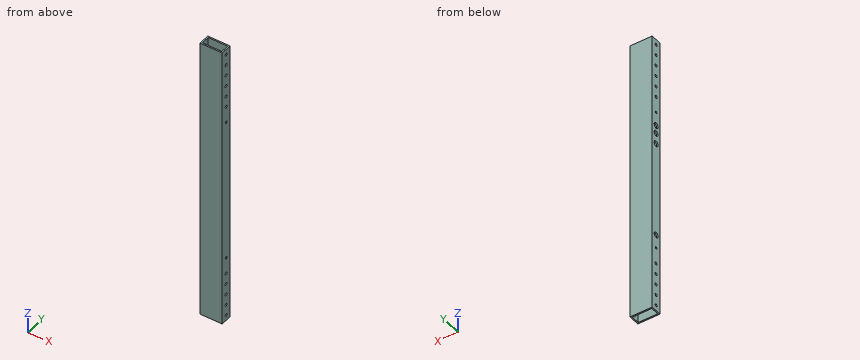
from build123d import *

# Parameters (mm, degrees)
BOSS_EXTRUDE1_DEPTH              = 330.2
BOSS_EXTRUDE1_DEPTH_BACK         = 330.2
SKETCH3_W                        = 50.8
SKETCH3_H                        = 25.4
SKETCH3_W_2                      = 44.45
SKETCH3_H_2                      = 19.05
F_1_4_0_25_DIAMETER_HOLE3_D      = 6.35
F_1_4_0_25_DIAMETER_HOLE4_D      = 6.35
F_1_4_0_25_DIAMETER_HOLE5_D      = 6.35
F_1_4_0_25_DIAMETER_HOLE6_D      = 6.35
F_1_4_0_25_DIAMETER_HOLE7_D      = 6.35
F_1_4_0_25_DIAMETER_HOLE8_D      = 6.35
F_13_64_0_20313_DIAMETER_HOLE1_D = 5.159502
F_1_2_0_5_DIAMETER_HOLE1_D       = 12.7
F_1_2_0_5_DIAMETER_HOLE1_DEPTH   = 6.35
F_1_2_0_5_DIAMETER_HOLE1_TIP     = 3.815464931


with BuildPart() as part:
    # Sketch3 → Boss-Extrude1 (new, two sides: drawn at the far end of the back side and taken through both)
    with BuildSketch(Plane.XY.offset(-BOSS_EXTRUDE1_DEPTH_BACK)):
        Rectangle(SKETCH3_W, SKETCH3_H)
        Rectangle(SKETCH3_W_2, SKETCH3_H_2, mode=Mode.SUBTRACT)
    extrude(amount=BOSS_EXTRUDE1_DEPTH + BOSS_EXTRUDE1_DEPTH_BACK)

    # 1/4 (0.25) Diameter Hole3 (through all)
    with Locations(Plane.ZY.offset(25.4)):
        with Locations((-317.5, 0)):
            Hole(F_1_4_0_25_DIAMETER_HOLE3_D / 2)

    # 1/4 (0.25) Diameter Hole4 (through all)
    with Locations(Plane.ZY.offset(25.4)):
        with Locations((292.1, 0), (317.5, 0)):
            Hole(F_1_4_0_25_DIAMETER_HOLE4_D / 2)

    # 1/4 (0.25) Diameter Hole5 (through all)
    with Locations(Plane(origin=(25.4, 0, 0), x_dir=(0, 0, -1), z_dir=(1, 0, 0))):
        with Locations((292.1, 0), (266.7, 0)):
            Hole(F_1_4_0_25_DIAMETER_HOLE5_D / 2)

    # 1/4 (0.25) Diameter Hole6 (through all)
    with Locations(Plane(origin=(25.4, 0, 0), x_dir=(0, 0, -1), z_dir=(1, 0, 0))):
        with Locations((215.9, 0), (241.3, 0)):
            Hole(F_1_4_0_25_DIAMETER_HOLE6_D / 2)

    # 1/4 (0.25) Diameter Hole7 (through all)
    with Locations(Plane(origin=(25.4, 0, 0), x_dir=(0, 0, -1), z_dir=(1, 0, 0))):
        with Locations((-190.5, 0), (-215.9, 0)):
            Hole(F_1_4_0_25_DIAMETER_HOLE7_D / 2)

    # 1/4 (0.25) Diameter Hole8 (through all)
    with Locations(Plane(origin=(25.4, 0, 0), x_dir=(0, 0, -1), z_dir=(1, 0, 0))):
        with Locations((-266.7, 0), (-241.3, 0)):
            Hole(F_1_4_0_25_DIAMETER_HOLE8_D / 2)

    # 13/64 (0.20313) Diameter Hole1 (through all)
    with Locations(Plane(origin=(25.4, 0, 0), x_dir=(0, 0, -1), z_dir=(1, 0, 0))):
        with Locations((-152.4, 0), (177.8, 0)):
            Hole(F_13_64_0_20313_DIAMETER_HOLE1_D / 2)

    # 1/2 (0.5) Diameter Hole1
    with Locations(Plane.ZY.offset(25.4)):
        with Locations((-146.050000508, 4.9e-08), (120.65, 1.7e-08), (101.600001492, 7.77e-07), (76.200001492, 7.03e-07)):
            Hole(F_1_2_0_5_DIAMETER_HOLE1_D / 2, depth=F_1_2_0_5_DIAMETER_HOLE1_DEPTH)
            with Locations((0, 0, -(F_1_2_0_5_DIAMETER_HOLE1_DEPTH + F_1_2_0_5_DIAMETER_HOLE1_TIP / 2))):  # 118° drill point
                Cone(0, F_1_2_0_5_DIAMETER_HOLE1_D / 2, F_1_2_0_5_DIAMETER_HOLE1_TIP, mode=Mode.SUBTRACT)


solid = part.part
The listing builds one solid part. Answer for the finished solid, in the listing's coordinates (mm). Coordinates: 2 decimals unless noted, no trailing zeros. Loops run counter-clockwise (first coordinate to the right, second up) from the corner with the lowest first, then second, coordinate; pieces in that order, holes last. Notation, with made-up numbers: (70.25, -12.75) -> (105.25, -12.75) arc R22 ccw to (105.25, 0.25) -> close; hole circle Ø7 at (4.5, 55). An arc over 180 degrees is marked (long way). Write item = value, one per line. Start each with the question number.
1) A cutting plane is placed at C-C (z = -146.05). Give the vertices of the cut face in (x, y) (3 decimals).
2) A cutting plane is placed at B-B (x = 0). Give the vertices of the cut face in (y, z) (3 decimals).
3) Straight lines are drawn through the part: line 1 (Y direction, x = -2, z = 264.5) (3 decimals); line 2 (X direction, y = -4.75, z = -74) (3 decimals); line 3 (Y direction, x = -24.55, z = -266.7) (3 decimals). For each, find the intervals that lie inside material, in ascending order. Write a range as from..to.
4) Given pin 1 Ø6 at (x, y) = (18.5, -5) entering from -Z, flat-ended and moving along its own axis, determine where the tip first touches the part or whether it passes through.
5) A cutting plane is placed at A-A (z = 173). Give the vertices of the cut face in (x, y) (3 decimals), then the cut area to 3 significant figures.
Responses:
q1.outline = (-25.4, -12.7) -> (25.4, -12.7) -> (25.4, 12.7) -> (-25.4, 12.7) -> (-25.4, 6.35) -> (-22.225, 6.35) -> (-22.225, 9.525) -> (22.225, 9.525) -> (22.225, -9.525) -> (-22.225, -9.525) -> (-22.225, -6.35) -> (-25.4, -6.35) -> close
q2.outline = (-12.7, -330.2) -> (-9.525, -330.2) -> (-9.525, 330.2) -> (-12.7, 330.2) -> close; (9.525, -330.2) -> (12.7, -330.2) -> (12.7, 330.2) -> (9.525, 330.2) -> close
q3.line_1 = -12.7..-9.525, 9.525..12.7
q3.line_2 = -25.4..-22.225, 22.225..25.4
q3.line_3 = -12.7..-3.175, 3.175..12.7
q4.pin_1 = through
q5.outline = (-25.4, -12.7) -> (25.4, -12.7) -> (25.4, 12.7) -> (-25.4, 12.7) -> close; hole (-22.225, -9.525) -> (22.225, -9.525) -> (22.225, 9.525) -> (-22.225, 9.525) -> close
q5.area = 444 mm²
